Read the model definition and answer for the solid it produces. Units are mm, in the model's axes. A direction names the side the tool comes from. Coordinates: 2 decimals unless noted, no trailing zeros. Loops run counter-clockwise (first coordinate to the right, second up) from the corner with the lowest first, then second, coordinate; pieces in that order, holes last.
from build123d import *

# Parameters (mm, degrees)
F1_DEPTH = 34.29
F3_R     = 31.75
F4_R     = 127
F5_R     = 19.05
F6_R     = 19.05
F7_T     = -5.08
F9_DEPTH = 2.54


with BuildPart() as f1:
    # F0 (on Front) → F1 (new body)
    with BuildSketch(Plane.XZ):
        Polygon((0, -193.235434227), (0, 48.064565773), (-30.48, 48.064565773), (-50.8, -23.055434227), (-25.4, -193.235434227), align=None)
    extrude(amount=F1_DEPTH)

    # F2: F1 across face


with BuildPart() as f1_1:
    add(f1.part)
    add(f1.part.mirror(Plane(origin=(0, -17.145, -72.585434227), x_dir=(0, 1, 0), z_dir=(1, 0, 0))))

    # F3
    f3_edges = [f1_1.edges().sort_by_distance(p)[0] for p in [
        (-30.48, -17.145, 48.064566),
        (30.48, -17.145, 48.064566),
    ]]
    fillet(f3_edges, radius=F3_R)

    # F4
    f4_edges = [f1_1.edges().sort_by_distance(p)[0] for p in [
        (-50.8, -17.145, -23.055434),
        (50.8, -17.145, -23.055434),
    ]]
    fillet(f4_edges, radius=F4_R)

    # F5
    f5_edges = [f1_1.edges().sort_by_distance(p)[0] for p in [
        (-25.4, -17.145, -193.235434),
        (25.4, -17.145, -193.235434),
    ]]
    fillet(f5_edges, radius=F5_R)

    # F6
    f6_edges = [f1_1.edges().sort_by_distance(p)[0] for p in [
        (37.282158, 0, -113.624977),
    ]]
    fillet(f6_edges, radius=F6_R)

    # F7
    f7_openings = [f1_1.faces().sort_by_distance(p)[0] for p in [
        (0, -34.29, -66.112083),
    ]]
    offset(amount=F7_T, openings=f7_openings)

    # F8 (on face) → F9 (join)
    with BuildSketch(Plane.XZ.offset(34.29)):
        with BuildLine():
            Line((6.530930145, 45.524565773), (-6.530930145, 45.524565773))
            ThreePointArc((-6.530930145, 45.524565773), (-24.121061084, 39.6343297845), (-34.6170446556, 24.3391699189))
            Line((-34.6170446556, 24.3391699189), (-40.8033894121, 2.6869632712))
            ThreePointArc((-40.8033894121, 2.6869632712), (-45.3287249612, -23.411952422), (-44.2285808171, -49.8774345649))
            Line((-44.2285808171, -49.8774345649), (-25.3113894552, -176.6226166898))
            ThreePointArc((-25.3113894552, -176.6226166898), (-19.7605371668, -186.6917922592), (-8.9822669545, -190.695434227))
            Line((-8.9822669545, -190.695434227), (8.9822669545, -190.695434227))
            ThreePointArc((8.9822669545, -190.695434227), (19.7605371668, -186.6917922592), (25.3113894552, -176.6226166898))
            Line((25.3113894552, -176.6226166898), (44.2285808171, -49.8774345649))
            ThreePointArc((44.2285808171, -49.8774345649), (45.3287249612, -23.411952422), (40.8033894121, 2.6869632712))
            Line((40.8033894121, 2.6869632712), (34.6170446556, 24.3391699189))
            ThreePointArc((34.6170446556, 24.3391699189), (24.121061084, 39.6343297845), (6.530930145, 45.524565773))
        make_face()
        with BuildLine():
            ThreePointArc((-32.1747738286, 23.641378254), (-22.5914844806, 37.6065242183), (-6.530930145, 42.984565773))
            Line((-6.530930145, 42.984565773), (6.530930145, 42.984565773))
            ThreePointArc((6.530930145, 42.984565773), (22.5914844806, 37.6065242183), (32.1747738286, 23.641378254))
            Line((32.1747738286, 23.641378254), (38.3611185851, 1.9891716064))
            ThreePointArc((38.3611185851, 1.9891716064), (42.7941003475, -23.5771131543), (41.7164081247, -49.5024834167))
            Line((41.7164081247, -49.5024834167), (22.7992167628, -176.2476655417))
            ThreePointArc((22.7992167628, -176.2476655417), (18.1023417495, -184.7677371773), (8.9822669545, -188.155434227))
            Line((8.9822669545, -188.155434227), (-8.9822669545, -188.155434227))
            ThreePointArc((-8.9822669545, -188.155434227), (-18.1023417495, -184.7677371773), (-22.7992167628, -176.2476655417))
            Line((-22.7992167628, -176.2476655417), (-41.7164081247, -49.5024834167))
            ThreePointArc((-41.7164081247, -49.5024834167), (-42.7941003475, -23.5771131543), (-38.3611185851, 1.9891716064))
            Line((-38.3611185851, 1.9891716064), (-32.1747738286, 23.641378254))
        make_face(mode=Mode.SUBTRACT)
    extrude(amount=F9_DEPTH)


solid = f1_1.part
Item 1: A cutting plane is placed at A-A on y = -28. Determine the outline of the cut face in (x, z).
Numbers:
outline: (-46.74, -50.25) - (-27.82, -177) arc R19.05 ccw to (-8.98, -193.24) - (8.98, -193.24) arc R19.05 ccw to (27.82, -177) - (46.74, -50.25) arc R127 ccw to (43.25, 3.38) - (37.06, 25.04) arc R31.75 ccw to (6.53, 48.06) - (-6.53, 48.06) arc R31.75 ccw to (-37.06, 25.04) - (-43.25, 3.38) arc R127 ccw to start; hole (-41.72, -49.5) - (-22.8, -176.25) arc R13.97 ccw to (-8.98, -188.16) - (8.98, -188.16) arc R13.97 ccw to (22.8, -176.25) - (41.72, -49.5) arc R121.92 ccw to (38.36, 1.99) - (32.17, 23.64) arc R26.67 ccw to (6.53, 42.98) - (-6.53, 42.98) arc R26.67 ccw to (-32.17, 23.64) - (-38.36, 1.99) arc R121.92 ccw to start
Item 2: Which of the six approach directions +Z, -Z, +X, -X, +Y, -Y give full straight-line access (tool end or side, diameter ignored) to faces 4 (the face through (45.352, -35.542, -23.783)), 5 (the face through (-32.125, -27.816, -113.762)), 6 (the face through (-23.9, -35.5, 39.8)), 7 (the face through (37.754, -35.542, 13.362))?
Numbers:
face 4: +X, -Y
face 5: -Y
face 6: +Z, -X, -Y
face 7: +Z, +X, -Y
Item 3: Find the intervals of material crossed by line 1 along Z through (x, y) = (-4.5, -31); line 2 along Y through (x, z) = (-4, -76.5); line 3 along X through (y, z) = (-15, -157), in increasing order.
Numbers:
line 1: z = -193.24 to -188.16, 42.98 to 48.06
line 2: y = -5.08 to 0
line 3: x = -30.37 to -25.07, 25.07 to 30.37
Item 4: Determine the mould class of faces 1 (the face through (0, -28, -188.155)), 2 (the face through (-37.67, -35.54, 13.66)), 3 (the face through (34.638, -35.542, -114.137)) for opening direction X: released by +X, released by -X, zero draft, split by the parting line, or undercut.
Numbers:
face 1: undercut
face 2: released by -X
face 3: released by +X
Item 5: A cutting plane is placed at B-B on x = 2. Determine the outline of the cut face in (y, z).
Numbers:
outline: (-36.83, -190.7) - (-34.29, -190.7) - (-34.29, -193.24) - (-19.05, -193.24) arc R19.05 ccw to (0, -174.19) - (0, 29.01) arc R19.05 ccw to (-19.05, 48.06) - (-34.29, 48.06) - (-34.29, 45.52) - (-36.83, 45.52) - (-36.83, 42.98) - (-19.05, 42.98) arc R13.97 cw to (-5.08, 29.01) - (-5.08, -174.19) arc R13.97 cw to (-19.05, -188.16) - (-36.83, -188.16) - close
Item 6: Given pin 1 (2 mm diameter, centred on x = -3.5, y = -35, fed in from -Z); pin 2 (3 mm diameter, centred on x = 24, y = -6, fed in from +Z); pin 3 (12 mm diameter, centred on x = -32.5, y = -31, fed in from -Z); pin 4 (10 mm diameter, centred on y = -5, z = -150.5, fed in from +X), each flat-ended and moving along its own axis, determine where each tip first touches the part or whether it passes through.
Numbers:
pin 1: stops at z = -193.24
pin 2: stops at z = 38.41
pin 3: stops at z = -181.67
pin 4: stops at x = 29.57
